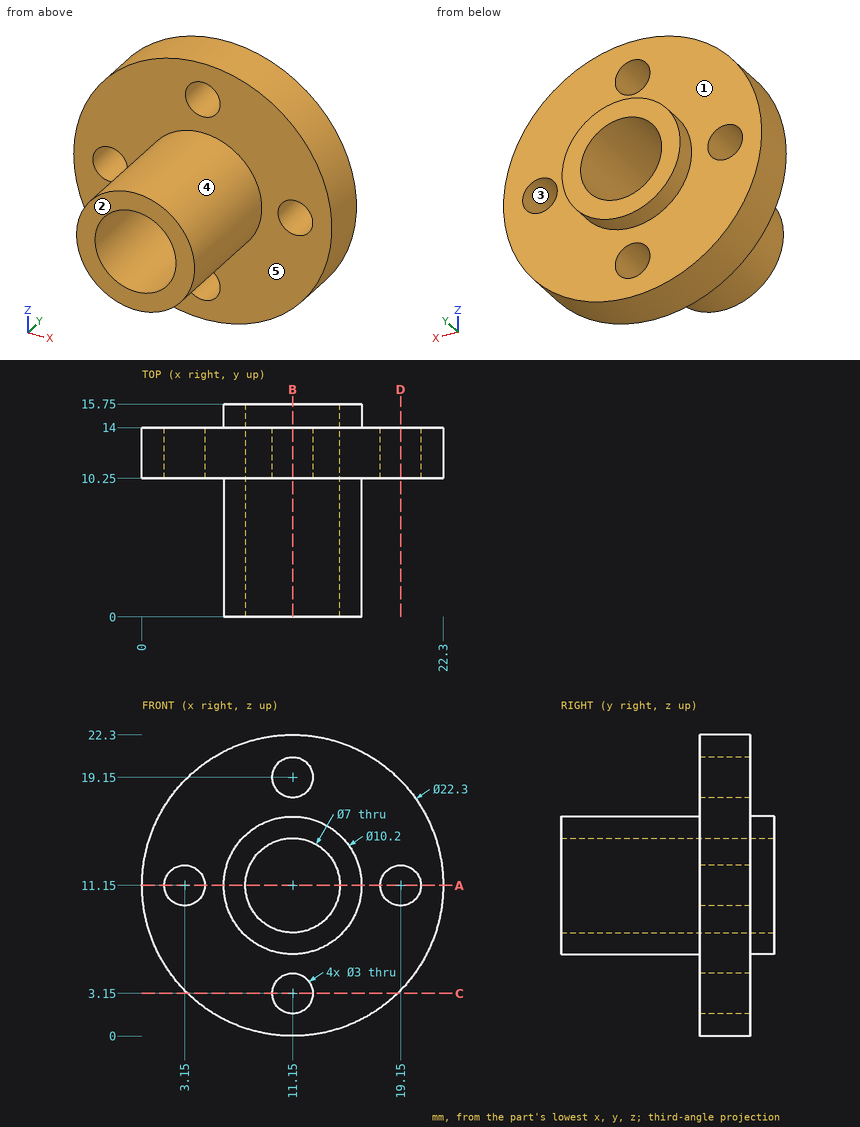
Here's the drawing with two shaded views (mm, measured from the low corner). I have some questions. A direction names the side the tool comes from. Give positions to 0.01 mm unless a question says otherwise; leave off trailing zeros. Loops run counter-clockwise (first coordinate to the right, second up) from the corner with the lowest first, then second, coordinate; pieces in that order, holes last. Notation, with made-up numbers: (-18, -36) -> (-14, -36) arc R15 cw to (-14, -29) -> close; hole circle Ø9 at (55.25, 15.5). An arc over 180 degrees is marked (long way). One line per item, written item: value.
Q1. I'm going to push flat-ended pins straight in: pin 1 Ø1.5 at (x, z) = (15, 18.5) entering from +Y; pin 2 Ø4 at (y, z) = (11, 19.5) entering from +X; pin 3 Ø2.5 at (x, z) = (19.15, 11.15) entering from -Y; pin 4 Ø1.5 at (y, z) = (3.5, 10.5) entering from -X. Where does each tip first touch, or does it pass through?
Answers follow:
pin 1: y = 14
pin 2: x = 20.32
pin 3: through
pin 4: x = 6.05
Q2. Suppose I cut it at B-B on x = 11.15. Please give me the cut outline in (y, z).
Answers follow:
outline: (0, 6.05) -> (10.25, 6.05) -> (10.25, 4.65) -> (14, 4.65) -> (14, 6.05) -> (15.75, 6.05) -> (15.75, 7.65) -> (0, 7.65) -> close; (0, 14.65) -> (15.75, 14.65) -> (15.75, 16.25) -> (14, 16.25) -> (14, 17.65) -> (10.25, 17.65) -> (10.25, 16.25) -> (0, 16.25) -> close; (10.25, 0) -> (14, 0) -> (14, 1.65) -> (10.25, 1.65) -> close; (10.25, 20.65) -> (14, 20.65) -> (14, 22.3) -> (10.25, 22.3) -> close
Q3. Suppose I cut it at D-D on x = 19.15. Please give me the cut outline in (y, z), then the cut area to 3 significant figures.
Answers follow:
outline: (10.25, 3.38) -> (14, 3.38) -> (14, 9.65) -> (10.25, 9.65) -> close; (10.25, 12.65) -> (14, 12.65) -> (14, 18.92) -> (10.25, 18.92) -> close
area: 47.0 mm^2
Q4. On a 3-axis mill with a long thin cutter (end or side, diameter ignored), from which of +Z, -Z, +X, -X, +Y, -Y can I reach the whole of each face in a straight line? I mean the marked faces 1 and 2. Say none if no direction works.
Answers follow:
face 1: +Y
face 2: +Z, -Z, +X, -X, -Y
Q5. If I drill on line 1 along Z through (x, y) = (11.15, 11.7); line 2 along Z through (x, y) = (11.15, 5.5); line 3 along Z through (x, y) = (12, 12.75), over which ranges is the centre line in solid material (lowest first)?
Answers follow:
line 1: 0 to 1.65, 4.65 to 7.65, 14.65 to 17.65, 20.65 to 22.3
line 2: 6.05 to 7.65, 14.65 to 16.25
line 3: 0.03 to 1.91, 4.39 to 7.75, 14.55 to 17.91, 20.39 to 22.27
Q6. Suppose I cut it at A-A on z = 11.15. Please give me the cut outline in (x, y).
Answers follow:
outline: (0, 10.25) -> (1.65, 10.25) -> (1.65, 14) -> (0, 14) -> close; (4.65, 10.25) -> (6.05, 10.25) -> (6.05, 0) -> (7.65, 0) -> (7.65, 15.75) -> (6.05, 15.75) -> (6.05, 14) -> (4.65, 14) -> close; (14.65, 0) -> (16.25, 0) -> (16.25, 10.25) -> (17.65, 10.25) -> (17.65, 14) -> (16.25, 14) -> (16.25, 15.75) -> (14.65, 15.75) -> close; (20.65, 10.25) -> (22.3, 10.25) -> (22.3, 14) -> (20.65, 14) -> close
Q7. Suppose I cut it at C-C on z = 3.15. Please give me the cut outline in (x, y).
Answers follow:
outline: (3.38, 10.25) -> (9.65, 10.25) -> (9.65, 14) -> (3.38, 14) -> close; (12.65, 10.25) -> (18.92, 10.25) -> (18.92, 14) -> (12.65, 14) -> close
Q8. We'd pull the mould along Z, two halves only. Please class the marked faces 3, 4 and 5: pulls with the +Z half, pulls with the -Z half, needs draft (parallel to the pull), parting line crosses it, or undercut.
Answers follow:
face 3: undercut
face 4: parting line crosses it
face 5: needs draft
